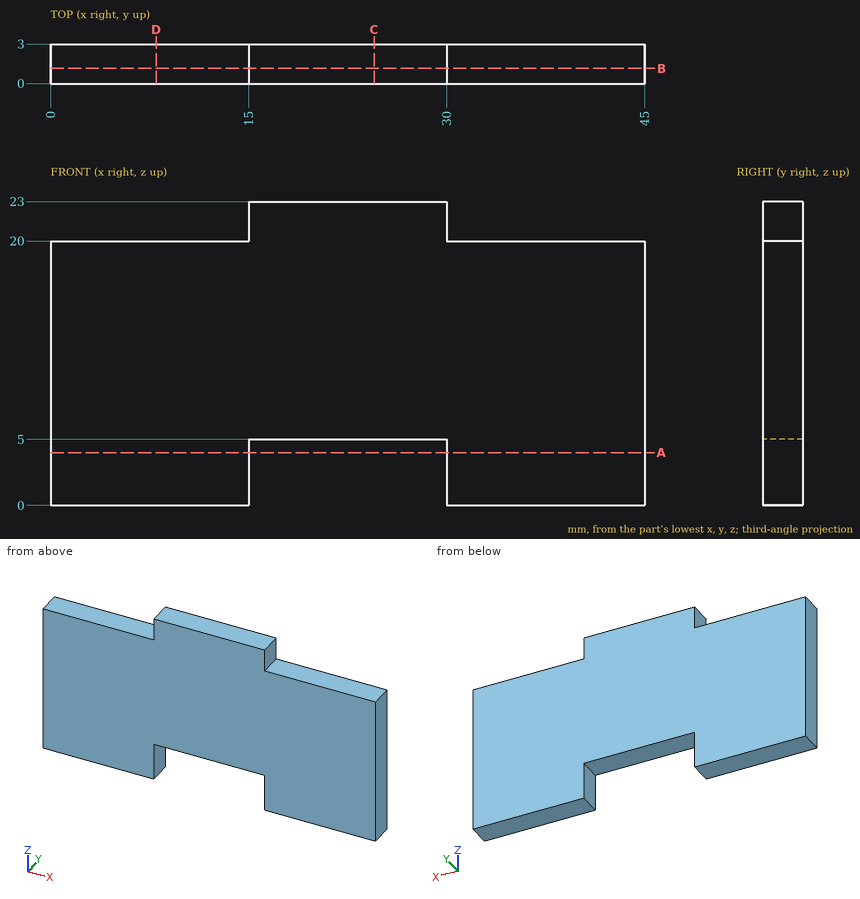
Part print with two shaded views. Sizes in mm from the minimum x, y, z corner. Round coordinates to 2 decimals unless told otherwise and drop trailing zeros. Loops run counter-clockwise (first coordinate to the right, second up) from the corner with the lowest first, then second, coordinate; pieces in that order, holes last. Notation, with made-up numbers: (41.5, 72.5) - (82.5, 72.5) arc R16 cw to (82.5, 99.5) - close; hole circle Ø4 at (5, -2). An arc over 180 degrees is marked (long way). Put each result on its own line as item: value.
1. Pin check, flat tips, straight feed: P1, Ø1.5, axis at x = 25, y = 2, coming from the -Z side; P2, Ø0.9, axis at y = 1, z = 21.5, coming from the -X side; P3, Ø0.9, axis at x = 35.5, y = 1.5, coming from the +Z side. Stop position of each tip, or through.
Geometry check:
P1: z = 5
P2: x = 15
P3: z = 20
2. Slice it at A-A on z = 4. List the corners of the cut face in (x, y), and give its area (3 significant figures).
Geometry check:
outline: (0, 0) - (15, 0) - (15, 3) - (0, 3) - close; (30, 0) - (45, 0) - (45, 3) - (30, 3) - close
area: 90.0 mm²
3. Slice it at D-D on x = 8. List the corners of the cut face in (y, z).
Geometry check:
outline: (0, 0) - (3, 0) - (3, 20) - (0, 20) - close
4. Slice it at C-C on x = 24.5. List the corners of the cut face in (y, z).
Geometry check:
outline: (0, 5) - (3, 5) - (3, 23) - (0, 23) - close
5. Wall check: line 1 (X direction, y = 1.05, z = 20.75); line 2 (Z direction, x = 30.5, y = 2.9); line 3 (Z direction, x = 17, y = 0.65). Give the ranges that are in metal, low to high.
Geometry check:
line 1: 15 to 30
line 2: 0 to 20
line 3: 5 to 23
6. Slice it at B-B on y = 1.15. List the corners of the cut face in (x, z).
Geometry check:
outline: (0, 0) - (15, 0) - (15, 5) - (30, 5) - (30, 0) - (45, 0) - (45, 20) - (30, 20) - (30, 23) - (15, 23) - (15, 20) - (0, 20) - close
